Design review of the part built by this model. Coordinates are the model's own, in mm. A direction names the side the tool comes from. Coordinates: 2 decimals unless noted, no trailing zeros. Loops run counter-clockwise (first coordinate to the right, second up) from the corner with the lowest first, then second, coordinate; pieces in that order, holes last. Notation, with made-up numbers: M 9,-35.5 L 64,-35.5 A20 cw 64,2.5 Z; hole C 14.25,26 d5. An arc over 180 degrees is marked long. Answer as a JSON object with one key per item and string values. Group by question number.
1. Insertion check: pin 1 (10 mm diameter, centred on x = 108.5, z = 55.5, fed in from -Y); pin 2 (8 mm diameter, centred on x = 93, y = 11.5, fed in from +Z); pin 3 (22 mm diameter, centred on x = 53.5, y = 42.5, fed in from -Z); pin 4 (1.5 mm diameter, centred on x = 59, y = 58.5, fed in from -Z). Each pin has a flat end and moves straight along its axis. Give the tip position at first contact, or say it passes through.
2. Draft analysis for pull direction Y (two halves, no side actions). For faces 1 (the flat face through (76, 60, 121)), 2 (the flat face through (130, 28, 103)), 3 (the flat face through (76, 58, 101)), state which applies: +Y half, -Y half, draft (parallel to the pull), parting line (faces both ways), or undercut.
3. To check wall thickness, follow probe 1 along Y at (x, z) = (130, 108.5); probe 2 along X at (y, z) = (20.5, 101); probe 3 along X at (y, z) = (21.5, 29.5). State the ranges of each line that lie inside material, in increasing order.
4. Consider section D-D (z = 56). State the section outline as (x, y) points, then the cut area to 3 significant figures.
5. Consider section C-C (x = 30.5). State the section outline as (y, z) points, then the cut area to 3 significant figures.
6. Consider section B-B (y = 8). State the section outline as (x, z) points.
7. Machinability: for faces 4 (the flat face through (108, 14, 103)), 5 (the flat face through (0, 16, 70)), 6 (the flat face through (59, 29, 80)), 7 (the flat face through (107, 15, 65)), which of the approach directions +Z, -Z, +X, -X, +Y, -Y give a long, thin tool a straight path to every point of the face, cutting with its end or side? Answer none if there is none.
8. Consider section A-A (z = 75). State the section outline as (x, y) points, then the cut area to 3 significant figures.
from build123d import *

# Parameters (mm, degrees)
BOX003_W     = 45
BOX003_H     = 27
BOX003_DEPTH = 75
BOX005_W     = 45
BOX005_H     = 27
BOX005_DEPTH = 75
BOX001_W     = 60
BOX001_H     = 27
BOX001_DEPTH = 140
BOX006_W     = 154
BOX006_H     = 31
BOX006_DEPTH = 5
BOX007_W     = 154
BOX007_H     = 5
BOX007_DEPTH = 40
BOX002_W     = 47
BOX002_H     = 29
BOX002_DEPTH = 76
BOX004_W     = 47
BOX004_H     = 29
BOX004_DEPTH = 76
BOX_W        = 62
BOX_H        = 29
BOX_DEPTH    = 141
FILLET_R     = 3


with BuildPart() as cube003:
    # Box003 → Box003 (new body)
    with BuildSketch(Plane(origin=(62, 1, 66), x_dir=(1, 0, 0), z_dir=(0, 0, 1))):
        with Locations((22.5, 13.5)):
            Rectangle(BOX003_W, BOX003_H)
    extrude(amount=BOX003_DEPTH)


with BuildPart() as cube005:
    # Box005 → Box005 (new body)
    with BuildSketch(Plane(origin=(108, 1, 66), x_dir=(1, 0, 0), z_dir=(0, 0, 1))):
        with Locations((22.5, 13.5)):
            Rectangle(BOX005_W, BOX005_H)
    extrude(amount=BOX005_DEPTH)


with BuildPart() as fusion001:
    # Box001 → Box001 (new body)
    with BuildSketch(Plane(origin=(1, 1, 1), x_dir=(1, 0, 0), z_dir=(0, 0, 1))):
        with Locations((30, 13.5)):
            Rectangle(BOX001_W, BOX001_H)
    extrude(amount=BOX001_DEPTH)

    # Fusion001: union Cube003, Cube005
    add(cube003.part)
    add(cube005.part)


with BuildPart() as cube006:
    # Box006 → Box006 (new body)
    with BuildSketch(Plane(origin=(0, 29, 136), x_dir=(1, 0, 0), z_dir=(0, 0, 1))):
        with Locations((77, 15.5)):
            Rectangle(BOX006_W, BOX006_H)
    extrude(amount=BOX006_DEPTH)


with BuildPart() as cube007:
    # Box007 → Box007 (new body)
    with BuildSketch(Plane(origin=(0, 55, 101), x_dir=(1, 0, 0), z_dir=(0, 0, 1))):
        with Locations((77, 2.5)):
            Rectangle(BOX007_W, BOX007_H)
    extrude(amount=BOX007_DEPTH)


with BuildPart() as cube002:
    # Box002 → Box002 (new body)
    with BuildSketch(Plane(origin=(61, 0, 65), x_dir=(1, 0, 0), z_dir=(0, 0, 1))):
        with Locations((23.5, 14.5)):
            Rectangle(BOX002_W, BOX002_H)
    extrude(amount=BOX002_DEPTH)


with BuildPart() as cube004:
    # Box004 → Box004 (new body)
    with BuildSketch(Plane(origin=(107, 0, 65), x_dir=(1, 0, 0), z_dir=(0, 0, 1))):
        with Locations((23.5, 14.5)):
            Rectangle(BOX004_W, BOX004_H)
    extrude(amount=BOX004_DEPTH)


with BuildPart() as fillet_body:
    # Box → Box (new body)
    with BuildSketch(Plane.XY):
        with Locations((31, 14.5)):
            Rectangle(BOX_W, BOX_H)
    extrude(amount=BOX_DEPTH)

    # Fusion: union Cube002, Cube004
    add(cube002.part)
    add(cube004.part)

    # Fusion002: union Cube006, Cube007
    add(cube006.part)
    add(cube007.part)

    # Cut: cut Fusion001
    add(fusion001.part, mode=Mode.SUBTRACT)

    # Fillet
    fillet_edges = [fillet_body.edges().sort_by_distance(p)[0] for p in [
        (77, 55, 136),
        (131, 29, 136),
        (84.5, 29, 136),
        (30.5, 29, 136),
    ]]
    fillet(fillet_edges, radius=FILLET_R)


solid = fillet_body.part
Findings below:
{
 "1": {"pin 1": "passes through", "pin 2": "stops at z = 66", "pin 3": "stops at z = 135.6", "pin 4": "stops at z = 101"},
 "2": {"face 1": "+Y half", "face 2": "undercut", "face 3": "draft"},
 "3": {"probe 1": "y = 0 to 1, 28 to 29, 55 to 60", "probe 2": "x = 0 to 1, 61 to 62, 107 to 108, 153 to 154", "probe 3": "x = 0 to 1, 61 to 62"},
 "4": {"outline": "M 0,0 L 62,0 L 62,29 L 0,29 Z; hole M 1,1 L 61,1 L 61,28 L 1,28 Z", "area": "178 mm^2"},
 "5": {"outline": "M 0,0 L 29,0 L 29,133 A3 cw 32,136 L 52,136 A3 cw 55,133 L 55,101 L 60,101 L 60,141 L 28,141 L 28,1 L 1,1 L 1,141 L 0,141 Z", "area": "643 mm^2"},
 "6": {"outline": "M 0,0 L 62,0 L 62,65 L 154,65 L 154,141 L 153,141 L 153,66 L 108,66 L 108,141 L 107,141 L 107,66 L 62,66 L 62,141 L 61,141 L 61,1 L 1,1 L 1,141 L 0,141 Z"},
 "7": {"face 4": "+Z", "face 5": "+Z, -Z, -X, +Y, -Y", "face 6": "-Z, +X, -X", "face 7": "-Z, +X, +Y, -Y"},
 "8": {"outline": "M 0,0 L 154,0 L 154,29 L 0,29 Z; hole M 1,1 L 61,1 L 61,28 L 1,28 Z; hole M 62,1 L 107,1 L 107,28 L 62,28 Z; hole M 108,1 L 153,1 L 153,28 L 108,28 Z", "area": "416 mm^2"}
}
